Answer from the drawing. Dimensions are ordinates in mm from the lowest x, y and z of the part. A direction names the side the tool comes from. Coordinates: 2 decimals unless noted, no trailing zeros. Write each loop counter-clockwise with the first axis right and the second up, starting at its lowest first coordinate (ties: lowest second). Pieces come first, ordered by that corner, then holes. Notation, with made-up numbers: (-39.5, 34) - (11.5, 34) arc R22 cw to (11.5, 71) - close; hole circle Ø4 at (8.5, 11.5). An arc over 180 degrees is marked (long way). Use a Markdown table: item, result.
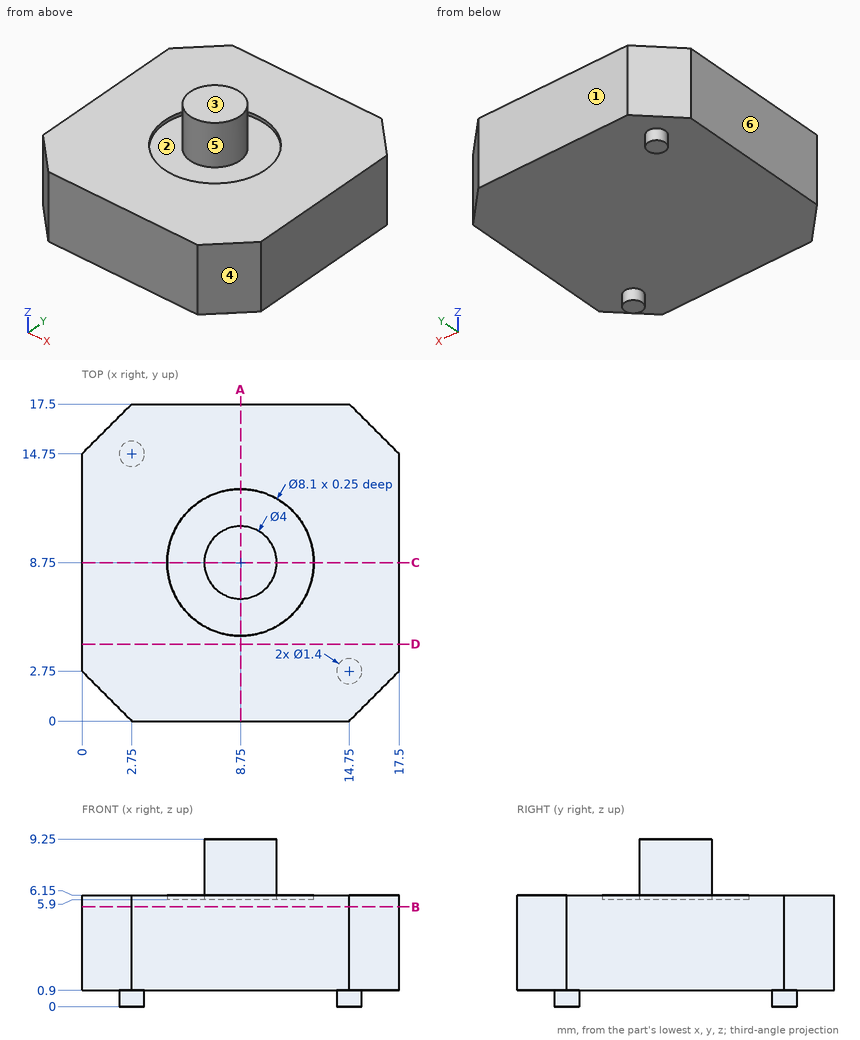
(1) For the marked faces 5 and 6, determine the directions among +Z, -Z, +X, -X, +Y, -Y from which every point of the face is accessible in a straight line to the end or side of a thin tool.
Report:
| item | result |
|---|---|
| face 5 | +Z |
| face 6 | +Z, -Z, -X, +Y, -Y |
(2) The mould has two halves that part along Y. Classify the marked faces 1, 2, 3 and 4: pulls with the +Y half, pulls with the -Y half, needs draft (parallel to the pull), parting line crosses it, or undercut.
Report:
| item | result |
|---|---|
| face 1 | pulls with the +Y half |
| face 2 | undercut |
| face 3 | needs draft |
| face 4 | pulls with the -Y half |
(3) Straight lines are drawn through the part: L1, parallel to Y at x = 8.75, z = 6.05; L2, parallel to Z at x = 12, y = 9.5; L3, parallel to Z at x = 16.5, y = 8. For each, find the intervals that lie inside material, in ascending order.
Report:
| item | result |
|---|---|
| L1 | y = 0 to 4.7, 6.75 to 10.75, 12.8 to 17.5 |
| L2 | z = 0.9 to 5.9 |
| L3 | z = 0.9 to 6.15 |
(4) A cutting plane is placed at B-B, the plane z = 5.5. Write down the section's boundary in (x, y), and give its area (3 significant figures).
Report:
| item | result |
|---|---|
| outline | (0, 2.75) - (2.75, 0) - (14.75, 0) - (17.5, 2.75) - (17.5, 14.75) - (14.75, 17.5) - (2.75, 17.5) - (0, 14.75) - close |
| area | 291 mm² |
(5) A cutting plane is placed at A-A, the plane x = 8.75. Write down the section's boundary in (y, z), and give its area (3 significant figures).
Report:
| item | result |
|---|---|
| outline | (0, 0.9) - (17.5, 0.9) - (17.5, 6.15) - (12.8, 6.15) - (12.8, 5.9) - (10.75, 5.9) - (10.75, 9.25) - (6.75, 9.25) - (6.75, 5.9) - (4.7, 5.9) - (4.7, 6.15) - (0, 6.15) - close |
| area | 103 mm² |
(6) Each of these flat-tipped pins is pushed along its axis until it touches: P1, Ø1, axis at x = 14, y = 3, coming from the +Z side; P2, Ø1, axis at x = 5.5, y = 6.5, coming from the -Z side; P3, Ø1, axis at y = 14, z = 7, coming from the +X side. Where does it stop, or does it pass through?
Report:
| item | result |
|---|---|
| P1 | stops at z = 6.15 |
| P2 | stops at z = 0.9 |
| P3 | passes through |
(7) A cutting plane is placed at D-D, the plane y = 4.25. Write down the section's boundary in (x, z).
Report:
| item | result |
|---|---|
| outline | (0, 0.9) - (17.5, 0.9) - (17.5, 6.15) - (0, 6.15) - close |
